Check sheet for the drawn part. Datum: minimum x, y, z corner. Units: mm. Coordinates: 2 decimals unless noted, no trailing zeros. Write each loop counter-clockwise with the first axis right and the second up, starting at its lowest first coordinate (ties: lowest second). Pieces come first, ordered by that corner, then holes. Notation, with made-up numbers: (29.5, -39.75) - (48.5, -39.75) arc R9 cw to (48.5, -27.75) - close; hole circle Ø5 at (72.25, 43.25). An arc over 180 degrees is marked (long way). Write each question's results on one line, items separated by ' | '.
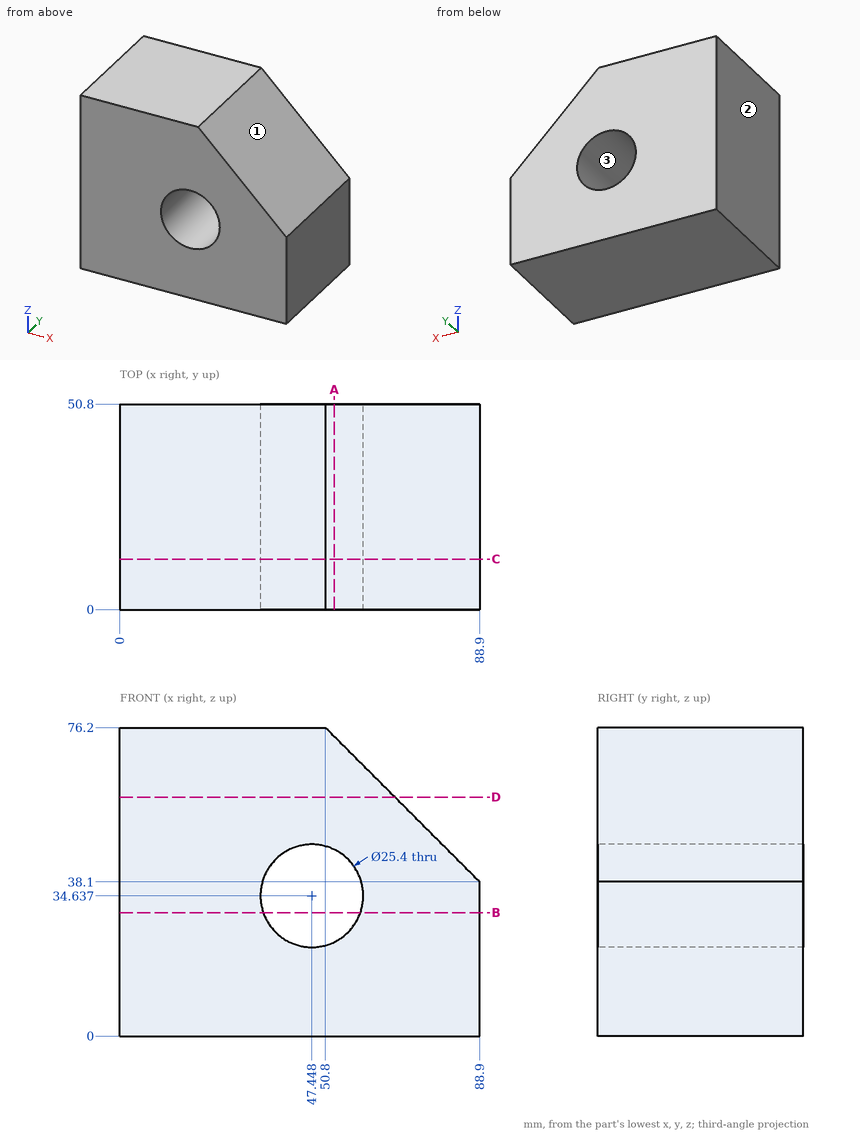
1. Sectioned sample at A-A (x = 53). Record the cut outline in (y, z) (1 decimal), then the cut area to 3 significant figures.
Values follow:
outline: (0, 0) - (50.8, 0) - (50.8, 23.2) - (0, 23.2) - close; (0, 46.1) - (50.8, 46.1) - (50.8, 74) - (0, 74) - close | area: 2,600 mm^2
2. Go/stop test with flat-tipped pins: pin 1 (2 mm diameter, centred on y = 9, z = 22.5, fed in from -X); pin 2 (20.5 mm diameter, centred on x = 47.45, z = 34.64, fed in from -Y). Record where each tip stops, or that it passes through.
Values follow:
pin 1: stops at x = 0 | pin 2: passes through
3. Sectioned sample at B-B (z = 30.5). Record the cut outline in (x, y) (1 decimal).
Values follow:
outline: (0, 0) - (35.4, 0) - (35.4, 50.8) - (0, 50.8) - close; (59.5, 0) - (88.9, 0) - (88.9, 50.8) - (59.5, 50.8) - close
4. Sectioned sample at C-C (y = 12.5). Record the cut outline in (x, z), then the cut area to 3 significant figures.
Values follow:
outline: (0, 0) - (88.9, 0) - (88.9, 38.1) - (50.8, 76.2) - (0, 76.2) - close; hole circle Ø25.4 at (47.45, 34.64) | area: 5,540 mm^2
5. Sectioned sample at D-D (z = 59). Record the cut outline in (x, y).
Values follow:
outline: (0, 0) - (68, 0) - (68, 50.8) - (0, 50.8) - close
6. Material ranges on L1, parallel to Z at x = 45, y = 26 (1 decimal); L2, parallel to X at y = 25, z = 42.5 (1 decimal); L3, parallel to Z at x = 41.5, y = 35 (1 decimal), recorded low to high. Write a range as [from, to].
Values follow:
L1: z = [0, 22.2], [47.1, 76.2] | L2: x = [0, 37.5], [57.4, 84.5] | L3: z = [0, 23.4], [45.9, 76.2]
7. Draft check along Z on the marked faces 1, 2 and 3. Enter one of: pulls with the +Z half, pulls with the -Z half, needs draft (parallel to the pull), parting line crosses it, or undercut.
Values follow:
face 1: pulls with the +Z half | face 2: needs draft | face 3: undercut
